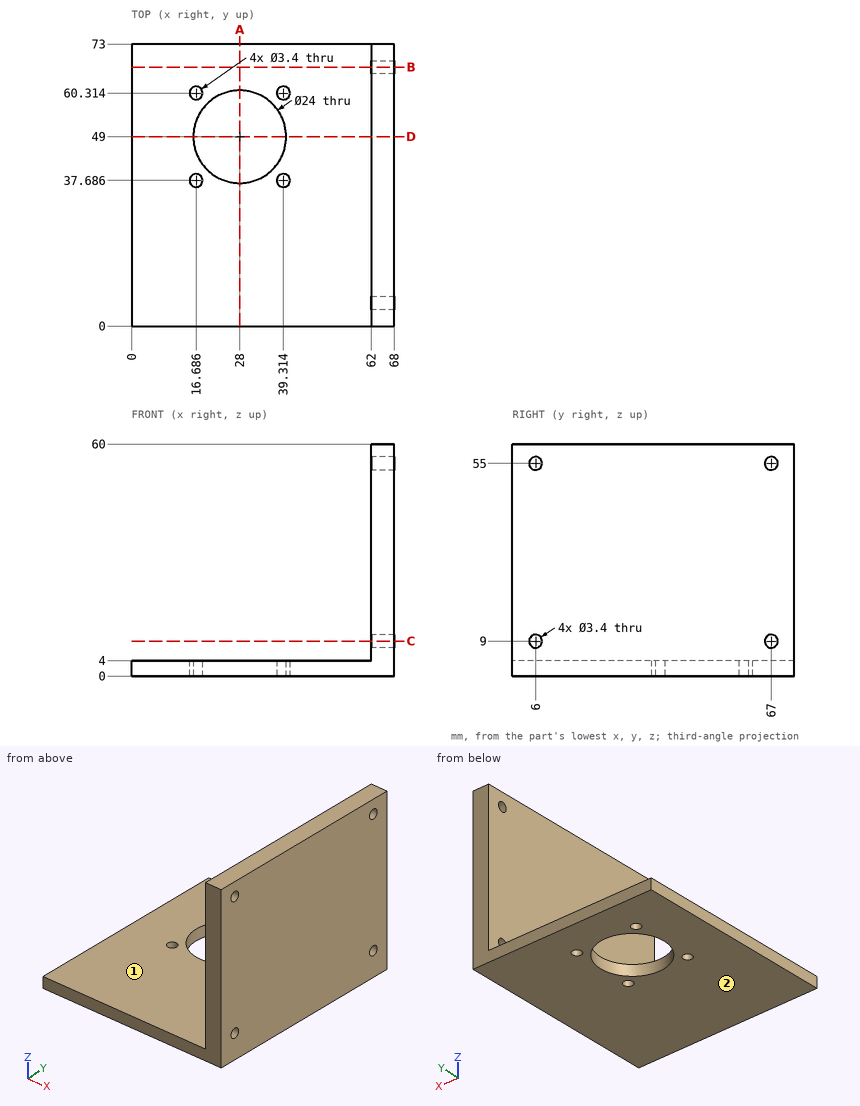
Job drawing, mm, ordinate dimensions from the low corner. One solid piece. A direction names the side the tool comes from. Coordinates: 2 decimals unless noted, no trailing zeros. Write each loop counter-clockwise with the first axis right and the second up, starting at its lowest first coordinate (ties: lowest second). Pieces come first, ordered by that corner, then holes. Notation, with made-up numbers: (87, 74.25) - (138, 74.25) arc R16 ccw to (138, 93.25) - close; hole circle Ø6 at (-35.5, 83). An arc over 180 degrees is marked (long way). Use a Markdown table: item, result. Add a question column.
Item 1: Flat gauge pins, fed straight in: pin 1 (5.5 mm diameter, centred on x = 39.31, y = 37.69, fed in from +Z); pin 2 (4 mm diameter, centred on x = 16.69, y = 60.31, fed in from -Z); pin 3 (2.5 mm diameter, centred on x = 39.31, y = 60.31, fed in from -Z); pin 4 (17 mm diameter, centred on y = 39.5, z = 42, fed in from -X). Where does each tip first touch, or does it go through?
Item 2: Drill centre lines: L1, parallel to X at y = 38, z = 3 (1 decimal); L2, parallel to X at y = 10.5, z = 26; L3, parallel to Z at x = 53, y = 14. Where is each one in solid material? Low to high. Write a range as from..to.
Item 3: Band-saw the part on C-C, the plane z = 9. Give the cut face in (x, y), and give its area (3 significant figures).
Item 4: Band-saw the part on B-B, the plane y = 67. Give the cut face in (x, z), and give its area (3 significant figures).
Item 5: Band-saw the part on D-D, the plane y = 49. Give the cut face in (x, z), and give its area (3 significant figures).
Item 6: Band-saw the part on A-A, the plane x = 28. Give the cut face in (y, z), and give its area (3 significant figures).
Item 7: 3-axis set-ups, long thin cutter, end or side, ignore diameter. For the marked faces 1 and 2: which of +Z, -Z, +X, -X, +Y, -Y reach the whole face in a straight line?
Numbers:
| question | item | result |
|---|---|---|
| 1 | pin 1 | z = 4 |
| 1 | pin 2 | z = 0 |
| 1 | pin 3 | through |
| 1 | pin 4 | x = 62 |
| 2 | L1 | 0..15, 18.4..23.2, 32.8..37.6, 41..68 |
| 2 | L2 | 62..68 |
| 2 | L3 | 0..4 |
| 3 | outline | (62, 0) - (68, 0) - (68, 4.3) - (62, 4.3) - close; (62, 7.7) - (68, 7.7) - (68, 65.3) - (62, 65.3) - close; (62, 68.7) - (68, 68.7) - (68, 73) - (62, 73) - close |
| 3 | area | 397 mm2 |
| 4 | outline | (0, 0) - (68, 0) - (68, 7.3) - (62, 7.3) - (62, 4) - (0, 4) - close; (62, 10.7) - (68, 10.7) - (68, 53.3) - (62, 53.3) - close; (62, 56.7) - (68, 56.7) - (68, 60) - (62, 60) - close |
| 4 | area | 567 mm2 |
| 5 | outline | (0, 0) - (16, 0) - (16, 4) - (0, 4) - close; (40, 0) - (68, 0) - (68, 60) - (62, 60) - (62, 4) - (40, 4) - close |
| 5 | area | 512 mm2 |
| 6 | outline | (0, 0) - (37, 0) - (37, 4) - (0, 4) - close; (61, 0) - (73, 0) - (73, 4) - (61, 4) - close |
| 6 | area | 196 mm2 |
| 7 | face 1 | +Z, -X, +Y, -Y |
| 7 | face 2 | -Z, +X, -X, +Y, -Y |
